Design review of the part built by this model. Coordinates are the model's own, in mm. Face numbers are marked on the shaded views. A direction names the side the tool comes from. Coordinates: 2 decimals unless noted, no trailing zeros. Loops run counter-clockwise (first coordinate to the right, second up) from the corner with the lowest first, then second, coordinate; pieces in that order, holes last. Notation, with made-up numbers: (27.5, 27) - (70.5, 27) arc R31 cw to (70.5, 51) - close; hole circle Ø11 at (85, 4). An arc over 180 degrees is marked (long way). One line per question, with ' | ' between items.
Autodesk Inventor part; units mm, degrees
ref_plane "YZ Plane" through (0, 0, 0) normal (1, 0, 0) x (0, 1, 0)
ref_plane "XZ Plane" through (0, 0, 0) normal (0, 1, 0) x (-1, 0, 0)
ref_plane "XY Plane" through (0, 0, 0) normal (0, 0, 1) x (1, 0, 0)
sketch "Sketch1" plane through (0, 0, 0) normal (0, 0, 1) x (1, 0, 0)
  line L0 (0, 0) -> (62.5, 0)
  line L1 (62.5, 0) -> (62.5, 66)
  line L2 (62.5, 66) -> (0, 66)
  line L3 (0, 66) -> (0, 0)
  dimension "d0" = 62.5
  dimension "d1" = 66
extrude "Extrusion1" add sketch "Sketch1" along normal blind 1.2
sketch "Sketch2" plane through (0, 0, 1.2) normal (0, 0, 1) x (1, 0, 0)
  line L0 (62.5, 66) -> (0, 66)
  line L1 (0, 66) -> (0, 0)
  line L2 (62.5, 66) -> (0, 66)
  line L3 (0, 66) -> (0, 64.4)
  line L4 (0, 64.4) -> (62.5, 64.4)
  line L5 (62.5, 64.4) -> (62.5, 66)
  line L6 (62.5, 0) -> (62.5, 66)
  line L7 (62.5, 0) -> (0, 0)
  line L8 (0, 0) -> (0, 1.6)
  line L9 (0, 1.6) -> (62.5, 1.6)
  line L10 (62.5, 1.6) -> (62.5, 0)
  line L11 (0, 0) -> (62.5, 0)
  line L12 (0, 66) -> (1.6, 66)
  line L13 (1.6, 66) -> (1.6, 0)
  line L14 (1.6, 0) -> (0, 0)
  line L15 (0, 0) -> (0, 66)
  line L16 (62.5, 64.4) -> (1.6, 64.4)
  line L17 (1.6, 64.4) -> (1.6, 1.6)
  line L18 (1.6, 1.6) -> (62.5, 1.6)
  line L19 (62.5, 1.6) -> (62.5, 64.4)
  dimension "d4" = 1.6
  dimension "d5" = 1.6
  dimension "d6" = 1.6
extrude "Extrusion2" add sketch "Sketch2" along normal blind 1.5 contours L6 L9 L13 L4
sketch "Sketch3" plane through (0, 0, 2.7) normal (0, 0, 1) x (1, 0, 0)
  line L0 (1.6, 1.6) -> (1.6, 64.4)
  line L1 (1.6, 1.6) -> (1.6, 64.4)
  line L2 (1.6, 33) -> (1.6, 43)
  line L3 (1.6, 43) -> (64.8797, 43)
  line L4 (64.8797, 43) -> (64.8797, 23)
  line L5 (64.8797, 23) -> (1.6, 23)
  line L6 (1.6, 23) -> (1.6, 43)
  point P0 (0, 0)
  point P1 (1.6, 23)
  dimension "d9" = 10
  dimension "d10" = 20
extrude "Extrusion3" cut sketch "Sketch3" against normal blind 1
sketch "Sketch4" plane through (0, 0, 2.7) normal (0, 0, 1) x (1, 0, 0)
  line L0 (62.5, 64.4) -> (1.6, 64.4)
  line L1 (62.5, 1.6) -> (1.6, 1.6)
  line L2 (1.6, 64.4) -> (60.9, 64.4)
  line L3 (60.9, 64.4) -> (60.9, 1.6)
  line L4 (60.9, 1.6) -> (1.6, 1.6)
  line L5 (1.6, 1.6) -> (1.6, 64.4)
  line L6 (0, 66) -> (0, 0)
  circle A0 centre (10, 56) radius 1.5
  line L7 (62.5, 0) -> (62.5, 66)
  circle A1 centre (52.5, 56) radius 1.5
  circle A2 centre (10, 10) radius 1.5
  circle A3 centre (52.5, 10) radius 1.5
  dimension "d13" = 59.3
extrude "Extrusion4" cut sketch "Sketch4" against normal through all contours A0 | A1 | A2 | A3
sketch "Sketch5" plane through (0, 0, 0) normal (0, 0, -1) x (-1, 0, 0)
  circle A0 centre (-52.5, 56) radius 1.5
  circle A1 centre (-52.5, 56) radius 6
  circle A2 centre (-10, 56) radius 1.5
  circle A3 centre (-10, 56) radius 6
  circle A4 centre (-52.5, 10) radius 1.5
  circle A5 centre (-52.5, 10) radius 6
  circle A6 centre (-10, 10) radius 1.5
  circle A7 centre (-10, 10) radius 6.5
  point P0 (0, 0)
  dimension "d22" = 12
  dimension "d23" = 12
  dimension "d24" = 12
  dimension "d25" = 13
extrude "Extrusion5" cut sketch "Sketch5" against normal blind 1.5 contours A0 | A1 | A3 | A4 | A5 | A7
fillet "Fillet1" radius 4 2 edges at (0, 66, 0.6) (0, 0, 0.6)
properties part number "SlaveLåg"
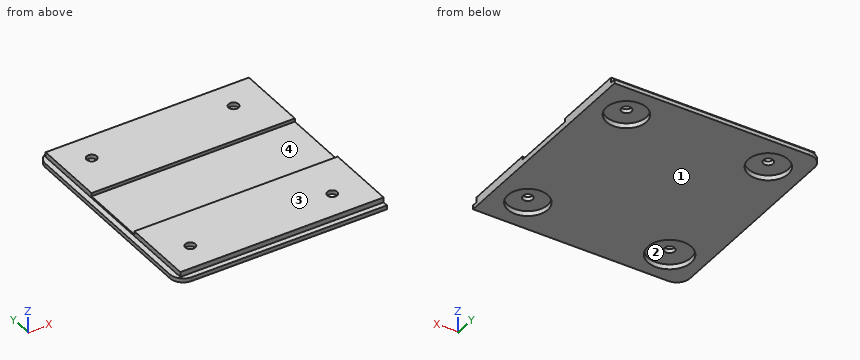
Q1. Take a section at B-B (z = 0.7). Give the boundary of the cut face in (x, y), plus the area to 3 significant figures.
Returned:
outline: (0, 4) arc R4 ccw to (4, 0) - (62.5, 0) - (62.5, 66) - (4, 66) arc R4 ccw to (0, 62) - close; hole circle Ø13 at (10, 10); hole circle Ø12 at (10, 56); hole circle Ø12 at (52.5, 10); hole circle Ø12 at (52.5, 56) | area: 3,650 mm²
Q2. Take a section at A-A (y = 10). Give the boundary of the cut face in (x, z).
Returned:
outline: (0, 0) - (3.5, 0) - (3.5, 1.5) - (8.5, 1.5) - (8.5, 2.7) - (1.6, 2.7) - (1.6, 1.2) - (0, 1.2) - close; (11.5, 1.5) - (16.5, 1.5) - (16.5, 0) - (46.5, 0) - (46.5, 1.5) - (51, 1.5) - (51, 2.7) - (11.5, 2.7) - close; (54, 1.5) - (58.5, 1.5) - (58.5, 0) - (62.5, 0) - (62.5, 2.7) - (54, 2.7) - close
Q3. Draft analysis for pull direction X (two halves, no side actions). For the marked faces 1 and 2, state which applies: +X half, -X half, draft (parallel to the pull), parting line (faces both ways), or undercut.
Returned:
face 1: draft | face 2: undercut
Q4. For pin 1 (0.8 mm diameter, centred on x = 31, z = 2, fed in from +Y); pin 2 (1 mm diameter, centred on x = 48, y = 56.5, fed in from -Z); pin 3 (0.5 mm diameter, centred on x = 23, z = 2, fed in from -Y), all flat-tipped, find the tip position at first contact; note any pin that passes through.
Returned:
pin 1: stops at y = 64.4 | pin 2: stops at z = 1.5 | pin 3: stops at y = 1.6
Q5. Take a section at D-D (y = 56). Give the boundary of the cut face in (x, z).
Returned:
outline: (0, 0) - (4, 0) - (4, 1.5) - (8.5, 1.5) - (8.5, 2.7) - (1.6, 2.7) - (1.6, 1.2) - (0, 1.2) - close; (11.5, 1.5) - (16, 1.5) - (16, 0) - (46.5, 0) - (46.5, 1.5) - (51, 1.5) - (51, 2.7) - (11.5, 2.7) - close; (54, 1.5) - (58.5, 1.5) - (58.5, 0) - (62.5, 0) - (62.5, 2.7) - (54, 2.7) - close
Q6. Tool access review of the marked faces 3 and 4: name each direction out of +Z, -Z, +X, -X, +Y, -Y from which nothing blocks a thin tool from reaching the whole face with its end or side.
Returned:
face 3: +Z, +X, -X, +Y, -Y | face 4: +Z, +X, -X
Q7. To check wall thickness, follow line 1 along Y through (x, z) = (10, 2.05); line 2 along Y through (x, z) = (56.5, 2.5); line 3 along X through (y, z) = (5, 1.65). State the ranges of each line that lie inside material, in increasing order.
Returned:
line 1: y = 1.6 to 8.5, 11.5 to 23, 43 to 54.5, 57.5 to 64.4 | line 2: y = 1.6 to 23, 43 to 64.4 | line 3: x = 1.6 to 62.5
Q8. Take a section at C-C (x = 33). Give the boundary of the cut face in (y, z).
Returned:
outline: (0, 0) - (66, 0) - (66, 1.2) - (64.4, 1.2) - (64.4, 2.7) - (43, 2.7) - (43, 1.7) - (23, 1.7) - (23, 2.7) - (1.6, 2.7) - (1.6, 1.2) - (0, 1.2) - close
